Part model, mm, in its own coordinate system. A direction names the side the tool comes from. Coordinates: 2 decimals unless noted, no trailing zeros. Order: outer loops, then holes, each group sorted by start corner. A loop starts at its lowest first (then second) coordinate and runs counter-clockwise, first axis right, second up.
```python
from build123d import *

# Parameters (mm, degrees)
SKETCH_1_W                  = 10
SKETCH_1_H                  = 42
CUT_EXTRUDE_4_DEPTH         = 72.414284285
CUT_EXTRUDE_4_DEPTH_BACK    = 72.414284285
SKETCH_7_R                  = 50
SKETCH_7_W                  = 60
SKETCH_7_H                  = 64
CUT_EXTRUDE_2_REACH         = 48.433
SKETCH_5_R                  = 2.1
PATTERN_CIRCULAR_1_COUNT    = 6
CUT_EXTRUDE_3_DEPTH         = 47.432747065
PATTERN_CIRCULAR_2_COUNT    = 4
HOLE_WIZARD_M61_D           = 5
HOLE_WIZARD_M61_DEPTH       = 17
HOLE_WIZARD_M61_CSINK_D     = 7
HOLE_WIZARD_M61_CSINK_ANGLE = 90
HOLE_WIZARD_M61_TIP         = 1.502151548
CHAMFER_1_SIZE              = 2
FILLET_1_R                  = 3


with BuildPart() as part:
    # Эскиз1 → Повернуть1 (revolve)
    with BuildSketch(Plane.XY, mode=Mode.PRIVATE) as revolve_1_sk:
        with Locations((5, 29)):
            Rectangle(SKETCH_1_W, SKETCH_1_H)
    revolve(revolve_1_sk.sketch.rotate(Axis((-29.36512031, 0, 0), (1, 0, 0)), 90), axis=Axis((-29.36512031, 0, 0), (1, 0, 0)))

    # Эскиз7 → Вырез-Вытянуть4 (cut, two sides: drawn at the far end of the back side and taken through both)
    with BuildSketch(Plane.ZY.offset(-CUT_EXTRUDE_4_DEPTH_BACK)):
        Circle(SKETCH_7_R)
        with Locations((0, 2)):
            Rectangle(SKETCH_7_W, SKETCH_7_H, mode=Mode.SUBTRACT)
    extrude(amount=CUT_EXTRUDE_4_DEPTH + CUT_EXTRUDE_4_DEPTH_BACK, mode=Mode.SUBTRACT)

    # Эскиз5 → Вырез-Вытянуть2 (cut, up to next)
    with BuildSketch(Plane.ZY, mode=Mode.PRIVATE) as cut_extrude_2_sk1:
        with Locations((0, 15)):
            Circle(SKETCH_5_R)
    cut_extrude_2_tool1 = extrude(cut_extrude_2_sk1.sketch, amount=-CUT_EXTRUDE_2_REACH, mode=Mode.PRIVATE) & part.part
    cut_extrude_2 = cut_extrude_2_tool1.solids().sort_by_distance((0, 15, 0))[0]
    add(cut_extrude_2, mode=Mode.SUBTRACT)

    # Круговой массив1: Вырез-Вытянуть2 ×6 about axis
    pattern_circular_1_axis = Axis((0, 0, 0), (1, 0, 0))
    for i in range(1, PATTERN_CIRCULAR_1_COUNT):
        add(cut_extrude_2.rotate(pattern_circular_1_axis, i * 360 / PATTERN_CIRCULAR_1_COUNT), mode=Mode.SUBTRACT)

    # Эскиз6 → Вырез-Вытянуть3 (cut, symmetric)
    with BuildSketch(Plane.ZY):
        with BuildLine():
            Line((-27.192031022, 24.222182541), (-25.777817459, 22.807968978))
            ThreePointArc((-25.777817459, 22.807968978), (-22.807968978, 22.807968978), (-22.807968978, 25.777817459))
            Line((-22.807968978, 25.777817459), (-24.222182541, 27.192031022))
            ThreePointArc((-24.222182541, 27.192031022), (-27.192031022, 27.192031022), (-27.192031022, 24.222182541))
        make_face()
    cut_extrude_3 = extrude(amount=CUT_EXTRUDE_3_DEPTH, both=True, mode=Mode.SUBTRACT)

    # Круговой массив2: Вырез-Вытянуть3 ×4 about axis
    pattern_circular_2_axis = Axis((0, 0, 0), (1, 0, 0))
    for i in range(1, PATTERN_CIRCULAR_2_COUNT):
        add(cut_extrude_3.rotate(pattern_circular_2_axis, i * 360 / PATTERN_CIRCULAR_2_COUNT), mode=Mode.SUBTRACT)

    # Отверстие обработанное метчиком M61
    with Locations(Plane(origin=(0, 34, 0), x_dir=(1, 0, 0), z_dir=(0, 1, 0))):
        with Locations((5, 15), (5, -15)):
            CounterSinkHole(HOLE_WIZARD_M61_D / 2, HOLE_WIZARD_M61_CSINK_D / 2, depth=HOLE_WIZARD_M61_DEPTH, counter_sink_angle=HOLE_WIZARD_M61_CSINK_ANGLE)
            with Locations((0, 0, -(HOLE_WIZARD_M61_DEPTH + HOLE_WIZARD_M61_TIP / 2))):  # 118° drill point
                Cone(0, HOLE_WIZARD_M61_D / 2, HOLE_WIZARD_M61_TIP, mode=Mode.SUBTRACT)

    # Фаска1
    chamfer_1_edges = [part.edges().sort_by_distance(p)[0] for p in [
        (0, 15, -2.1),
        (0, 9.318653348, 11.940381057),
        (0, -5.681346652, 14.040381057),
        (0, -15, 2.1),
        (0, -9.318653348, -11.940381057),
        (0, 5.681346652, -14.040381057),
    ]]
    chamfer(chamfer_1_edges, length=CHAMFER_1_SIZE)

    # Скругление1
    fillet_1_edges = [part.edges().sort_by_distance(p)[0] for p in [
        (5, 34, -30),
        (5, 34, 30),
        (5, -30, 30),
        (5, -30, -30),
    ]]
    fillet(fillet_1_edges, radius=FILLET_1_R)


solid = part.part
```
(1) Slice it at A-A, the plane y = 0. Give the cut face in (x, z), then the cut area to 3 significant figures.
(2) Drop a flat-ended pin along its axis: pin 1 (6.5 mm diameter, centred on y = -7.5, z = -12.99, fed in from -X). Give the stop position or say it passes through.
(3) Probe line 1 (Y direction, x = 9.25, z = -13); line 2 (Y direction, x = 7.25, z = 0); line 3 (Z direction, x = 5, y = 28.5). List the from-to ranges inside material, lowest first.
(4) Pull direction Z, two halves, no side cores. Call faces 1 (the face through (4.566, 15.759, -15.019)), 2 (the face through (4.93, 33.1, -29.14)), 3 (the face through (4.68, 15.759, 14.707)), 4 (the face through (10, 9, 0)): +Z half, -Z half, draft (parallel to the pull), parting line (faces both ways), or undercut.
(5) Slice it at C-C, the plane x = 4.25. State how many separate pieces and enclosed holes the cut face has, then the cut area to 3 significant figures.
(6) Slice it at B-B, the plane z = 0. Give the cut face in (x, y).
(7) Tool access for faces 5 (the face through (5, -30, 0)), 6 (the face through (2.69, 24.89, 15.96)), 7 (the face through (4.93, 26.49, 23.52)): list every direction of +Z, -Z, +X, -X, +Y, -Y with a clear straight run to the whole face (end or side of a thin tool).
Here are the results:
1. outline: (0, -30) - (10, -30) - (10, -8) - (0, -8) - close; (0, 8) - (10, 8) - (10, 30) - (0, 30) - close
1. area: 440 mm2
2. pin 1: stops at x = 0.85
3. line 1: y = -30 to -9.6, -5.4 to 5.4, 9.6 to 34
3. line 2: y = -30 to -17.1, -12.9 to -8, 8 to 12.9, 17.1 to 34
3. line 3: z = -30 to -17.5, -12.5 to 12.5, 17.5 to 30
4. face 1: undercut
4. face 2: -Z half
4. face 3: undercut
4. face 4: draft
5. separate pieces: 1
5. enclosed holes: 11
5. area: 3,290 mm2
6. outline: (0, -30) - (10, -30) - (10, -17.1) - (2, -17.1) - (0, -19.1) - close; (0, -10.9) - (2, -12.9) - (10, -12.9) - (10, -8) - (0, -8) - close; (0, 8) - (10, 8) - (10, 12.9) - (2, 12.9) - (0, 10.9) - close; (0, 19.1) - (2, 17.1) - (10, 17.1) - (10, 34) - (0, 34) - close
7. face 5: +Z, -Z, +X, -X, -Y
7. face 6: +Y
7. face 7: +X, -X
